Job drawing, mm, ordinate dimensions from the low corner. One solid piece. A direction names the side the tool comes from. Give positions to 0.01 mm unless a question says otherwise; leave off trailing zeros. Write each loop counter-clockwise with the first axis right and the second up, starting at its lowest first coordinate (ties: lowest second). Pieces come first, ordered by that corner, then holes. Notation, with made-up numbers: (-8, -9) - (26, -9) arc R22 cw to (26, 10) - close; hole circle Ø9 at (-25.5, 50). An arc over 180 degrees is marked (long way). Answer as a JSON object with one key per item and string values.
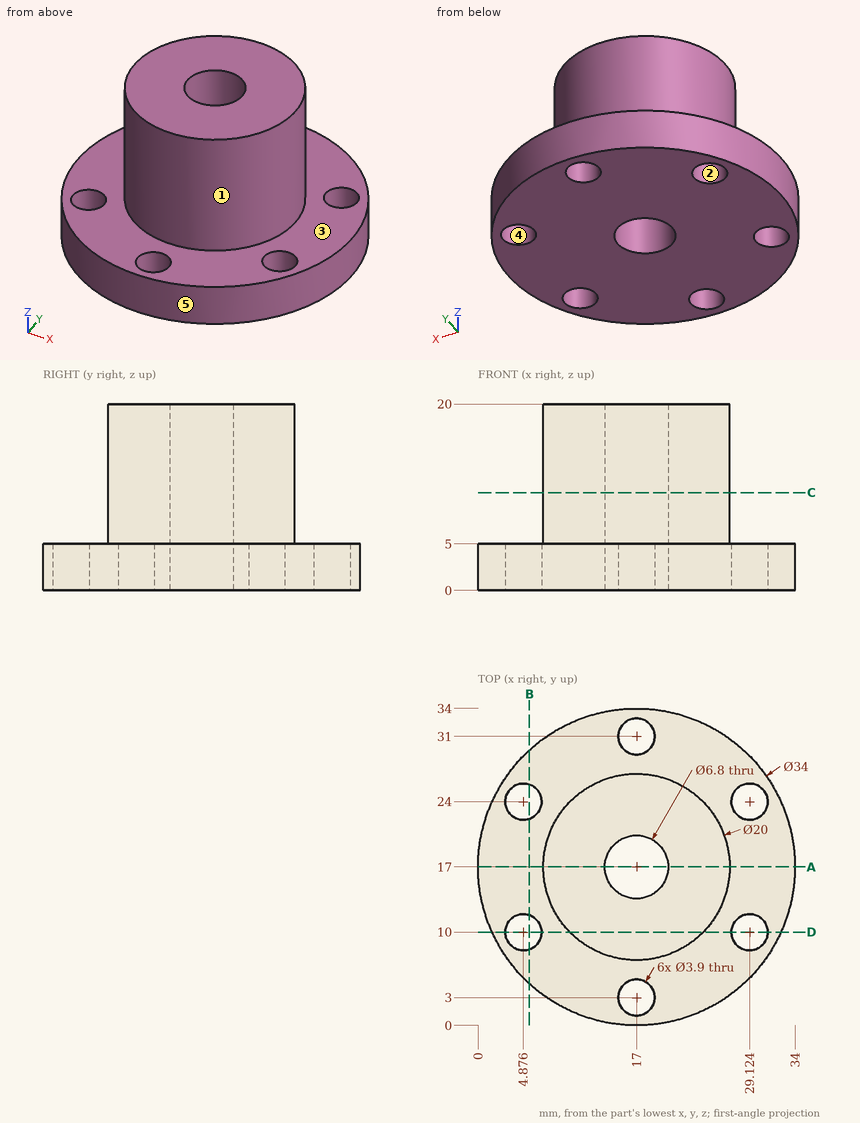
Item 1: Cut at D-D (y = 10). Give the cut face in (x, z) (1 decimal).
Entries:
{"outline": "(1.5, 0) - (2.9, 0) - (2.9, 5) - (1.5, 5) - close; (6.8, 0) - (27.2, 0) - (27.2, 5) - (24.1, 5) - (24.1, 20) - (9.9, 20) - (9.9, 5) - (6.8, 5) - close; (31.1, 0) - (32.5, 0) - (32.5, 5) - (31.1, 5) - close"}
Item 2: Cut at C-C (z = 10.5). Give the cut face in (x, y).
Entries:
{"outline": "circle Ø20 at (17, 17); hole circle Ø6.8 at (17, 17)"}
Item 3: Which spindle directions (+Z, -Z, +X, -X, +Y, -Y) get a long thin tool onto all of the face, cutting with end or side? Do the marked faces 1 and 2. Say none if no direction does.
Entries:
{"face 1": "+Z", "face 2": "+Z, -Z"}
Item 4: Cut at A-A (y = 17). Give the cut face in (x, z).
Entries:
{"outline": "(0, 0) - (13.6, 0) - (13.6, 20) - (7, 20) - (7, 5) - (0, 5) - close; (20.4, 0) - (34, 0) - (34, 5) - (27, 5) - (27, 20) - (20.4, 20) - close"}
Item 5: Cut at B-B (x = 5.5). Give the cut face in (y, z).
Entries:
{"outline": "(4.48, 0) - (8.15, 0) - (8.15, 5) - (4.48, 5) - close; (11.85, 0) - (22.15, 0) - (22.15, 5) - (11.85, 5) - close; (25.85, 0) - (29.52, 0) - (29.52, 5) - (25.85, 5) - close"}
Item 6: Probe line 1 (Y direction, x = 17, z = 1.1); line 2 (X direction, y = 24, z = 3.55) (1 decimal); line 3 (Y direction, x = 17, z = 15). List the from-to ranges inside material, lowest first. Write a range as from..to.
Entries:
{"line 1": "0..1.05, 4.95..13.6, 20.4..29.05, 32.95..34", "line 2": "1.5..2.9, 6.8..27.2, 31.1..32.5", "line 3": "7..13.6, 20.4..27"}
Item 7: Mould opens along Y. For the marked faces 3, 4 and 5 say: +Y half, -Y half, draft (parallel to the pull), parting line (faces both ways), or undercut.
Entries:
{"face 3": "draft", "face 4": "undercut", "face 5": "parting line"}
Item 8: Flat gauge pins, fed straight in: P1, Ø3, axis at x = 26, z = 16.5, coming from the -Y side (1 decimal); P2, Ø5, axis at y = 18, z = 10.5, coming from the +X side; P3, Ø3, axis at x = 17, y = 3, coming from the -Z side; P4, Ø5, axis at x = 17, y = 31, coming from the +Z side. Where does each tip first touch, or does it go through?
Entries:
{"P1": "y = 10.4", "P2": "x = 27", "P3": "through", "P4": "z = 5"}
